Can you work these out from the model? Positions are in its coordinate system, mm. Give positions to 0.01 mm unless a question says otherwise; leave off trailing zeros. Order: outer loops, then holes, each group sorted by start corner. A loop starts at its lowest first (then second) coordinate and runs counter-clockwise, first axis right, second up. Notation, with made-up numbers: (-38.75, -6) -> (-12.75, -6) arc R18 cw to (-12.75, 16) -> close; hole circle Ø9 at (61, -10.5). An arc over 180 degrees is marked (long way). Answer as a JSON object with one key per item and string values.
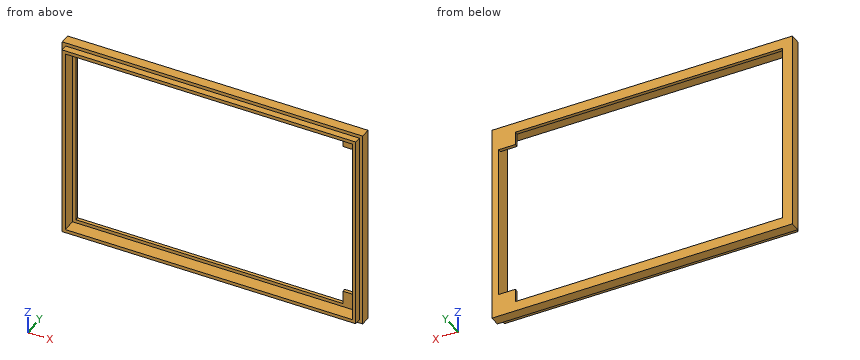
```python
from build123d import *

# Parameters (mm, degrees)
SKETCH1_W           = 90
SKETCH1_H           = 61
SKETCH1_W_2         = 86
SKETCH1_H_2         = 57
BOSS_EXTRUDE1_DEPTH = 3
BOSS_EXTRUDE2_DEPTH = 1
SKETCH3_W           = 88
SKETCH3_H           = 59
SKETCH3_W_2         = 86
SKETCH3_H_2         = 57
BOSS_EXTRUDE3_DEPTH = 2


with BuildPart() as part:
    # Sketch1 → Boss-Extrude1 (new body)
    with BuildSketch(Plane(origin=(0, 0, 0), x_dir=(1, 0, 0), z_dir=(0, 1, 0))):
        with Locations((45, 30.5)):
            Rectangle(SKETCH1_W, SKETCH1_H)
        with Locations((45, 30.5)):
            Rectangle(SKETCH1_W_2, SKETCH1_H_2, mode=Mode.SUBTRACT)
    extrude(amount=BOSS_EXTRUDE1_DEPTH)

    # Sketch2 → Boss-Extrude2 (add)
    with BuildSketch(Plane(origin=(0, 3, 0), x_dir=(1, 0, 0), z_dir=(0, 1, 0))):
        Polygon((88, 59), (83, 59), (3, 59), (2, 59), (2, 2), (3, 2), (83, 2), (88, 2), (88, 7), (83, 7), (83, 3), (3, 3), (3, 58), (83, 58), (83, 54), (88, 54), align=None)
    extrude(amount=-BOSS_EXTRUDE2_DEPTH)

    # Sketch3 → Boss-Extrude3 (add)
    with BuildSketch(Plane.XZ):
        with Locations((45, -30.5)):
            Rectangle(SKETCH3_W, SKETCH3_H)
        with Locations((45, -30.5)):
            Rectangle(SKETCH3_W_2, SKETCH3_H_2, mode=Mode.SUBTRACT)
    extrude(amount=BOSS_EXTRUDE3_DEPTH)


solid = part.part
```
1. If we section it at A-A on z = -35.5: Please give me the cut outline in (x, y).
Worked answers:
{"outline": "(0, 0) -> (1, 0) -> (1, -2) -> (2, -2) -> (2, 2) -> (3, 2) -> (3, 3) -> (0, 3) -> close; (88, -2) -> (89, -2) -> (89, 0) -> (90, 0) -> (90, 3) -> (88, 3) -> close"}
2. Please list where these lines run through material, in increasing order: L1, parallel to Z at x = 80.5, y = -0.9; L2, parallel to X at y = 0.3, z = -46; L3, parallel to Z at x = 48, y = 1.
Worked answers:
{"L1": "-60 to -59, -2 to -1", "L2": "0 to 2, 88 to 90", "L3": "-61 to -59, -2 to 0"}
3. Will these pins go through, and if not, where does the flat tip stop? pin 1 Ø1.6 at (y, z) = (-1, -41.5) entering from -X; pin 2 Ø0.6 at (y, z) = (-1, -39.5) entering from +X; pin 3 Ø2 at (x, y) = (64, -1.5) entering from -Z.
Worked answers:
{"pin 1": "x = 1", "pin 2": "x = 89", "pin 3": "z = -60"}
4. If we section it at C-C on x = 36: Please give me the cut outline in (y, z).
Worked answers:
{"outline": "(-2, -60) -> (0, -60) -> (0, -61) -> (3, -61) -> (3, -58) -> (2, -58) -> (2, -59) -> (-2, -59) -> close; (-2, -2) -> (2, -2) -> (2, -3) -> (3, -3) -> (3, 0) -> (0, 0) -> (0, -1) -> (-2, -1) -> close"}
5. If we section it at B-B on y = 1.05: Please give me the cut outline in (x, z), then the cut area to 3 significant figures.
Worked answers:
{"outline": "(0, -61) -> (90, -61) -> (90, 0) -> (0, 0) -> close; hole (2, -59) -> (88, -59) -> (88, -2) -> (2, -2) -> close", "area": "588 mm²"}
